Can you work these out from the model? Positions are in its coordinate system, mm. A direction names the side the tool comes from. Coordinates: 2 decimals unless noted, no trailing zeros. Order: outer loops, then holes, each group sorted by start corner. A loop starts at its lowest first (then second) coordinate and runs counter-clockwise, first axis right, second up. Notation, with made-up numbers: (50, -36.75) - (82, -36.75) arc R15 cw to (82, -18.75) - close; hole circle Ø4 at (45.5, 50.5). An arc over 180 degrees is marked (long way). Use a Markdown table: item, result. Add a question column.
(1) I want a section at A-A (z = 187.5). List the corners of the cut face in (x, y) for me (3 decimals), and give its area (3 significant figures).
(2) If I drill on L1, parallel to Y at x = 6, z = 444 (3 decimals); L2, parallel to X at y = -16.5, z = 183 (3 decimals); L3, parallel to Z at x = 1.75, y = -17, over which ranges is the centre line in solid material (lowest first)? Write a range as [from, to].
(3) I want a section at C-C (x = 17.75). List the corners of the cut face in (y, z) for me (3 decimals).
(4) For pin 1 Ø23 at (y, z) = (-25.4, 411.72) entering from +X, with a flat end and sliding along its axis, tell me the tip position at first contact or that it passes through.
(5) I want a section at B-B (z = 38.1). List the corners of the cut face in (x, y) for me (1 decimal), and give its area (3 significant figures).
(6) We'd pull the mould along Y, two halves only. Please class faces 1 (the flat face through (13, 0, 276)), 2 (the cylindrical face through (1.61, -21.11, 398.09)), 3 (the cylindrical face through (1.61, -24.77, 230.98)), 4 (the flat face through (13, -50.8, 276)): pulls with the +Y half, pulls with the -Y half, needs draft (parallel to the pull), parting line crosses it, or undercut.
(7) I want a section at D-D (y = -25.4). State how many separate pieces and enclosed holes the cut face has, and give its area (3 significant figures).
(8) On a 3-axis mill with a long thin cutter (end or side, diameter ignored), from which of +Z, -Z, +X, -X, +Y, -Y can I reach the whole of each face in a straight line? I mean faces 5 (the flat face through (13, -3.175, 276)), 6 (the cylindrical face through (1.6, -21.1, 134.5)). Say none if no direction works.
Autodesk Inventor part; units mm, degrees
ref_plane "YZ Plane" through (0, 0, 0) normal (1, 0, 0) x (0, 1, 0)
ref_plane "XZ Plane" through (0, 0, 0) normal (0, 1, 0) x (-1, 0, 0)
ref_plane "XY Plane" through (0, 0, 0) normal (0, 0, 1) x (1, 0, 0)
sketch "Sketch1" plane through (0, 0, 0) normal (0, 0, 1) x (1, 0, 0)
  line L0 (0, 0) -> (25.4, 0)
  line L1 (25.4, 0) -> (25.4, -50.8)
  line L2 (25.4, -50.8) -> (0, -50.8)
  line L3 (0, -50.8) -> (0, 0)
  line L4 (22.225, -3.175) -> (3.175, -3.175)
  line L5 (3.175, -3.175) -> (3.175, -47.625)
  line L6 (3.175, -47.625) -> (22.225, -47.625)
  line L7 (22.225, -47.625) -> (22.225, -3.175)
  dimension "d0" = 25.4
  dimension "d1" = 50.8
  dimension "d2" = 3.175
extrude "Extrusion1" add sketch "Sketch1" along normal blind 559.8439
sketch "Sketch2" plane through (25.4, -50.8, 0) normal (1, 0, 0) x (0, 0, -1)
  circle A0 centre (-38.1, 25.4) radius 14.2875
  circle A1 centre (-148.1252, 25.4) radius 14.2875
  line L0 (0, 50.8) -> (0, 0)
  line L1 (-559.8439, 0) -> (-559.8439, 50.8)
  line L2 (0, 50.8) -> (-559.8439, 50.8)
  line L3 (0, 0) -> (-559.8439, 0)
  circle A2 centre (-216.7052, 25.4) radius 14.2875
  dimension "d7" = 25.4
  dimension "d8" = 25.4
  dimension "d9" = 28.575
  dimension "d10" = 28.575
  dimension "d14" = 110.0252
  dimension "d15" = 38.1
  dimension "d24" = 68.58
  dimension "d25" = 28.575
  dimension "d26" = 25.4
extrude "Extrusion2" cut sketch "Sketch2" against normal blind 254 contours A0 | A1
sketch "Sketch3" plane through (25.4, -50.8, 0) normal (1, 0, 0) x (0, 0, -1)
  circle A0 centre (-521.7439, 25.4) radius 14.2875
  circle A1 centre (-411.7188, 25.4) radius 14.2875
  line L0 (-559.8439, 0) -> (-559.8439, 50.8)
  line L1 (0, 50.8) -> (-559.8439, 50.8)
  dimension "d16" = 38.1
  dimension "d17" = 110.0252
  dimension "d18" = 25.4
  dimension "d19" = 25.4
  dimension "d20" = 28.575
  dimension "d21" = 28.575
extrude "Extrusion3" cut sketch "Sketch3" against normal blind 25.4
sketch "Sketch4" plane through (25.4, -50.8, 0) normal (1, 0, 0) x (0, 0, -1)
  circle A0 centre (-216.7052, 25.4) radius 14.2875
  circle A1 centre (-148.1252, 25.4) radius 14.2875
  line L0 (0, 0) -> (-559.8439, 0)
  point P0 (0, 50.8)
  dimension "d27" = 68.58
  dimension "d28" = 28.575
  dimension "d29" = 25.4
extrude "Extrusion4" cut sketch "Sketch4" against normal blind 25.4 contours A0
properties part number "DRL Short"
Answers follow:
| question | item | result |
|---|---|---|
| 1 | outline | (0, -50.8) - (25.4, -50.8) - (25.4, 0) - (0, 0) - close; hole (3.175, -47.625) - (22.225, -47.625) - (22.225, -3.175) - (3.175, -3.175) - close |
| 1 | area | 444 mm² |
| 2 | L1 | y = [-50.8, -47.625], [-3.175, 0] |
| 2 | L2 | x = [0, 3.175], [22.225, 25.4] |
| 2 | L3 | z = [0, 26.54], [49.66, 136.57], [159.68, 205.15], [228.26, 400.16], [423.28, 510.19], [533.3, 559.84] |
| 3 | outline | (-50.8, 0) - (-47.625, 0) - (-47.625, 559.844) - (-50.8, 559.844) - close; (-3.175, 0) - (0, 0) - (0, 559.844) - (-3.175, 559.844) - close |
| 4 | pin 1 | passes through |
| 5 | outline | (0, -50.8) - (25.4, -50.8) - (25.4, -39.7) - (22.2, -39.7) - (22.2, -47.6) - (3.2, -47.6) - (3.2, -39.7) - (0, -39.7) - close; (0, -11.1) - (3.2, -11.1) - (3.2, -3.2) - (22.2, -3.2) - (22.2, -11.1) - (25.4, -11.1) - (25.4, 0) - (0, 0) - close |
| 5 | area | 262 mm² |
| 6 | face 1 | pulls with the +Y half |
| 6 | face 2 | undercut |
| 6 | face 3 | undercut |
| 6 | face 4 | pulls with the -Y half |
| 7 | separate pieces | 12 |
| 7 | enclosed holes | 0 |
| 7 | area | 2,650 mm² |
| 8 | face 5 | +Z, -Z |
| 8 | face 6 | +X, -X |
